Read the model definition and answer for the solid it produces. Units are mm, in the model's axes. Give positions to 0.01 mm unless a question says otherwise; leave off trailing zeros. Order: outer loops, then holes, each group sorted by start corner. A loop starts at its lowest first (then second) coordinate and runs counter-clockwise, first axis right, second up. Notation, with made-up numbers: (68.5, 1) - (122.5, 1) arc R15 ccw to (122.5, 14) - close; hole circle Ø5 at (23, 17). An arc over 180 degrees is marked (long way). Write each question's results on one line, items separated by ' | '. Start each with the question number.
Q1. Find section C-C on x = -13. Give the vertices of the cut face in (y, z), and give its area (3 significant figures).
Q2. Find section B-B on z = 49.5. Give the vertices of the cut face in (x, y).
Q3. Find section A-A on y = 27. Give the vertices of the cut face in (x, z), and give its area (3 significant figures).
Q4. Find the intervals of material crossed by line 1 along X through (y, z) = (30, -51); line 2 along X through (y, z) = (46.5, 241.5); line 3 along Y through (x, z) = (-32, 173), in increasing order. Write a range as from..to.
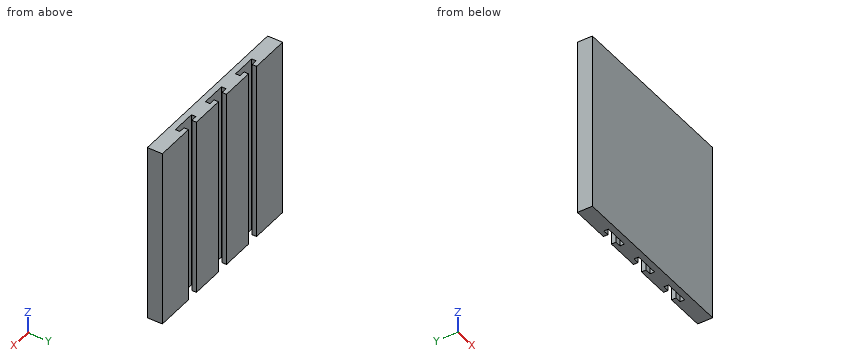
Autodesk Inventor part; units mm, degrees
ref_plane "YZ Plane" through (0, 0, 0) normal (1, 0, 0) x (0, 1, 0)
ref_plane "XZ Plane" through (0, 0, 0) normal (0, 1, 0) x (-1, 0, 0)
ref_plane "XY Plane" through (0, 0, 0) normal (0, 0, 1) x (1, 0, 0)
sketch "Sketch1" plane through (0, 0, 0) normal (0, 0, 1) x (1, 0, 0)
  line L0 (-300, 0) -> (300, 0)
  line L1 (300, 0) -> (300, 50)
  line L2 (-300, 50) -> (-300, 0)
  line L3 (-20, 50) -> (-20, 35)
  line L4 (-20, 35) -> (-40, 35)
  line L5 (-40, 35) -> (-40, 20)
  line L6 (-40, 20) -> (40, 20)
  line L7 (40, 20) -> (40, 35)
  line L8 (40, 35) -> (20, 35)
  line L9 (20, 35) -> (20, 50)
  line L10 (-75, 159.793) -> (-75, -97.8722) construction
  line L11 (75, 159.793) -> (75, -92.8199) construction
  line L12 (-130, 50) -> (-130, 35)
  line L13 (-130, 35) -> (-110, 35)
  line L14 (-110, 35) -> (-110, 20)
  line L15 (-110, 20) -> (-190, 20)
  line L16 (-190, 20) -> (-190, 35)
  line L17 (-190, 35) -> (-170, 35)
  line L18 (-170, 35) -> (-170, 50)
  line L19 (170, 50) -> (170, 35)
  line L20 (170, 35) -> (190, 35)
  line L21 (190, 35) -> (190, 20)
  line L22 (190, 20) -> (110, 20)
  line L23 (110, 20) -> (110, 35)
  line L24 (110, 35) -> (130, 35)
  line L25 (130, 35) -> (130, 50)
  line L26 (-20, 50) -> (-130, 50)
  line L27 (-170, 50) -> (-300, 50)
  line L28 (300, 50) -> (170, 50)
  line L29 (130, 50) -> (20, 50)
  point P0 (0, 0)
  dimension "d0" = 300
  dimension "d1" = 600
  dimension "d2" = 50
  dimension "d3" = 50
  dimension "d4" = 20
  dimension "d5" = 20
  dimension "d6" = 20
  dimension "d7" = 20
  dimension "d8" = 30
  dimension "d9" = 15
  dimension "d10" = 15
  dimension "d12" = 75
  dimension "d13" = 75
  dimension "d14" = 15
  dimension "d15" = 109.793
  dimension "d16" = 142.8199
  dimension "d17" = 109.793
  dimension "d18" = 147.8722
extrude "Extrusion1" add sketch "Sketch1" along normal mid plane 600
properties part number "base plate"
Working result:
1) outline: (0, -300) - (20, -300) - (20, 300) - (0, 300) - close | area: 12,000 mm²
2) outline: (-300, 0) - (300, 0) - (300, 50) - (170, 50) - (170, 35) - (190, 35) - (190, 20) - (110, 20) - (110, 35) - (130, 35) - (130, 50) - (20, 50) - (20, 35) - (40, 35) - (40, 20) - (-40, 20) - (-40, 35) - (-20, 35) - (-20, 50) - (-130, 50) - (-130, 35) - (-110, 35) - (-110, 20) - (-190, 20) - (-190, 35) - (-170, 35) - (-170, 50) - (-300, 50) - close
3) outline: (-300, -300) - (-190, -300) - (-190, 300) - (-300, 300) - close; (-110, -300) - (-40, -300) - (-40, 300) - (-110, 300) - close; (40, -300) - (110, -300) - (110, 300) - (40, 300) - close; (190, -300) - (300, -300) - (300, 300) - (190, 300) - close | area: 216,000 mm²
4) line 1: -300..-190, -110..-40, 40..110, 190..300 | line 2: -300..-170, -130..-20, 20..130, 170..300 | line 3: 0..20, 35..50
